CAD build for the part. Positions are in the model's coordinates, mm. A direction names the side the tool comes from. Round coordinates to 2 decimals unless told otherwise and drop trailing zeros. Loops run counter-clockwise (first coordinate to the right, second up) from the corner with the lowest first, then second, coordinate; pieces in that order, holes last.
from build123d import *

# Parameters (mm, degrees)
SKETCH1_R           = 7
SKETCH1_R_2         = 5
SKETCH1_R_3         = 10
BOSS_EXTRUDE1_DEPTH = 15


with BuildPart() as part:
    # Sketch1 → Boss-Extrude1 (new, symmetric)
    with BuildSketch(Plane.XY):
        with BuildLine():
            ThreePointArc((-18.313197236, -27.452264151), (-10.929939867, -36.447383635), (-9.804034884, -48.03))
            ThreePointArc((-9.804034884, -48.03), (0, -60), (9.804034884, -48.03))
            ThreePointArc((9.804034884, -48.03), (10.929939867, -36.447383635), (18.313197236, -27.452264151))
            ThreePointArc((18.313197236, -27.452264151), (19.978209416, -26.265398313), (21.566520754, -24.9776937))
            ThreePointArc((21.566520754, -24.9776937), (30.697148757, -22.889346352), (37.550915036, -29.273345896))
            ThreePointArc((37.550915036, -29.273345896), (54.555971575, -32.550365911), (48.899852708, -16.182130593))
            ThreePointArc((48.899852708, -16.182130593), (38.43354311, -10.563553249), (33, 0))
            ThreePointArc((33, 0), (31.461859707, 9.957478785), (26.990825227, 18.986715186))
            ThreePointArc((26.990825227, 18.986715186), (17.541357446, 39.155919937), (15.576262231, 61.342124263))
            ThreePointArc((15.576262231, 61.342124263), (15.761817989, 63.174110312), (16, 65))
            ThreePointArc((16, 65), (0, 81), (-16, 65))
            ThreePointArc((-16, 65), (-15.761817989, 63.174110312), (-15.576262231, 61.342124263))
            ThreePointArc((-15.576262231, 61.342124263), (-17.541357446, 39.155919937), (-26.990825227, 18.986715186))
            ThreePointArc((-26.990825227, 18.986715186), (-31.461859707, 9.957478785), (-33, 0))
            ThreePointArc((-33, 0), (-38.43354311, -10.563553249), (-48.899852708, -16.182130593))
            ThreePointArc((-48.899852708, -16.182130593), (-54.555971575, -32.550365911), (-37.550915036, -29.273345896))
            ThreePointArc((-37.550915036, -29.273345896), (-30.697148757, -22.889346352), (-21.566520754, -24.9776937))
            ThreePointArc((-21.566520754, -24.9776937), (-19.978209416, -26.265398313), (-18.313197236, -27.452264151))
        make_face()
        with Locations((-47, -26)):
            Circle(SKETCH1_R, mode=Mode.SUBTRACT)
        with Locations((0, -50)):
            Circle(SKETCH1_R_2, mode=Mode.SUBTRACT)
        with BuildLine():
            ThreePointArc((19.1, -5.93211598), (17.320508076, -10), (14.687363137, -13.575027222))
            ThreePointArc((14.687363137, -13.575027222), (7, -12.124355653), (4.412636863, -19.507143202))
            ThreePointArc((4.412636863, -19.507143202), (0, -20), (-4.412636863, -19.507143202))
            ThreePointArc((-4.412636863, -19.507143202), (-7, -12.124355653), (-14.687363137, -13.575027222))
            ThreePointArc((-14.687363137, -13.575027222), (-17.320508076, -10), (-19.1, -5.93211598))
            ThreePointArc((-19.1, -5.93211598), (-14, 0), (-19.1, 5.93211598))
            ThreePointArc((-19.1, 5.93211598), (-17.320508076, 10), (-14.687363137, 13.575027222))
            ThreePointArc((-14.687363137, 13.575027222), (-7, 12.124355653), (-4.412636863, 19.507143202))
            ThreePointArc((-4.412636863, 19.507143202), (0, 20), (4.412636863, 19.507143202))
            ThreePointArc((4.412636863, 19.507143202), (7, 12.124355653), (14.687363137, 13.575027222))
            ThreePointArc((14.687363137, 13.575027222), (17.320508076, 10), (19.1, 5.93211598))
            ThreePointArc((19.1, 5.93211598), (14, 0), (19.1, -5.93211598))
        make_face(mode=Mode.SUBTRACT)
        with Locations((47, -26)):
            Circle(SKETCH1_R, mode=Mode.SUBTRACT)
        with Locations((0, 65)):
            Circle(SKETCH1_R_3, mode=Mode.SUBTRACT)
    extrude(amount=BOSS_EXTRUDE1_DEPTH, both=True)


solid = part.part
Item 1: Cut at D-D (x = 45.5). List the corners of the cut face in (y, z), plus the area to 3 significant figures.
Verdict:
outline: (-35.89, -15) - (-32.84, -15) - (-32.84, 15) - (-35.89, 15) - close; (-19.16, -15) - (-15.21, -15) - (-15.21, 15) - (-19.16, 15) - close
area: 210 mm2
Item 2: Cut at C-C (z = 2). State how many separate pieces and enclosed holes the cut face has, plus the area to 3 significant figures.
Verdict:
separate pieces: 1
enclosed holes: 5
area: 4,900 mm2
Item 3: Cut at A-A (x = 0). List the corners of the cut face in (y, z).
Verdict:
outline: (-60, -15) - (-55, -15) - (-55, 15) - (-60, 15) - close; (-45, -15) - (-20, -15) - (-20, 15) - (-45, 15) - close; (20, -15) - (55, -15) - (55, 15) - (20, 15) - close; (75, -15) - (81, -15) - (81, 15) - (75, 15) - close
Item 4: Mould opens along X. For faces 4 (the cylindrical face through (0, -60, 0)), 5 (the cylindrical face through (50.23, -32.21, -0.21)), 6 (the cylindrical face through (-38.316, -10.443, 0.21)) say: released by +X, released by -X, zero draft, split by the parting line, or undercut.
Verdict:
face 4: split by the parting line
face 5: undercut
face 6: released by -X
Item 5: Wall check: L1, parallel to Y at x = 0, z = -0.75; L2, parallel to X at y = -24, z = 9; L3, parallel to Y at x = 5.5, z = 0.75. Give the ranges that are in metal, low to high.
Verdict:
L1: y = -60 to -55, -45 to -20, 20 to 55, 75 to 81
L2: x = -56.8 to -53.71, -40.29 to -33.29, -22.91 to 22.91, 33.29 to 40.29, 53.71 to 56.8
L3: y = -58.35 to -13.35, 13.35 to 56.65, 73.35 to 80.02
Item 6: Flat gauge pins, fed straight in: P1, Ø8, axis at y = 66.5, z = -8, coming from the +X side; P2, Ø2, axis at x = 33.5, z = 12, coming from the -Y side; P3, Ø4, axis at x = 9, z = -10, coming from the -Y side; P4, Ø8.5, axis at x = 47, y = -26, coming from the +Z side. Where does each tip first touch, or does it go through?
Verdict:
P1: stops at x = 16
P2: stops at y = -24.86
P3: stops at y = -57.14
P4: passes through
Item 7: Cut at B-B (x = -47). List the corners of the cut face in (y, z), plus the area to 3 significant figures.
Verdict:
outline: (-36, -15) - (-33, -15) - (-33, 15) - (-36, 15) - close; (-19, -15) - (-15.72, -15) - (-15.72, 15) - (-19, 15) - close
area: 188 mm2
Item 8: 3-axis set-ups, long thin cutter, end or side, ignore diameter. For faces 1 (the cylindrical face through (-31.42, 10.09, 0.21)), 2 (the cylindrical face through (10.867, -36.6, 0.21)), 3 (the cylindrical face through (19.96, -26.28, 0.21)): which of +Z, -Z, +X, -X, +Y, -Y reach the whole face in a straight line?
Verdict:
face 1: +Z, -Z, -X, +Y
face 2: +Z, -Z
face 3: +Z, -Z, -Y
